```python
from build123d import *

# Parameters (mm, degrees)
SKETCH_1_W      = 40
SKETCH_1_H      = 40
EXTRUDE_1_DEPTH = 20
SKETCH_2_R      = 3
EXTRUDE_2_DEPTH = 4.5
SKETCH_4_R      = 2
SKETCH_4_W      = 8
SKETCH_4_H      = 20
EXTRUDE_4_DEPTH = 2.7
SKETCH_5_W      = 4
SKETCH_5_H      = 7
EXTRUDE_5_DEPTH = 7


with BuildPart() as part:
    # 草图1 → 凸台-拉伸1 (new body)
    with BuildSketch(Plane(origin=(0, 0, 0), x_dir=(1, 0, 0), z_dir=(0, 1, 0))):
        with Locations((20, 20)):
            Rectangle(SKETCH_1_W, SKETCH_1_H)
    extrude(amount=EXTRUDE_1_DEPTH)

    # 草图2 → 凸台-拉伸2 (add)
    with BuildSketch(Plane.XY):
        with Locations(Location((10, 10, 0), (0, 0, 180))):
            Circle(SKETCH_2_R)
    extrude(amount=EXTRUDE_2_DEPTH)

    # 草图4 → 凸台-拉伸4 (add)
    # profile 1 of 3: a face of its own
    with BuildSketch(Plane(origin=(0, 0, -12.3), x_dir=(-1, 0, 0), z_dir=(0, 0, -1))):
        with BuildLine():
            Line((-44.5, 17), (-44.5, 20))
            Line((-44.5, 20), (-48, 20))
            Line((-48, 20), (-48, 0))
            Line((-48, 0), (-40, 0))
            Line((-40, 0), (-40, 15))
            Line((-40, 15), (-42.5, 15))
            ThreePointArc((-42.5, 15), (-45.914213562, 13.585786438), (-44.5, 17))
        make_face()
        with Locations((-44.5, 5)):
            Circle(SKETCH_4_R, mode=Mode.SUBTRACT)
    # profile 2 of 3: a face of its own
    with BuildSketch(Plane(origin=(0, 0, -12.3), x_dir=(-1, 0, 0), z_dir=(0, 0, -1))):
        with BuildLine():
            Line((-40, 15), (-40, 20))
            Line((-40, 20), (-44.5, 20))
            Line((-44.5, 20), (-44.5, 17))
            ThreePointArc((-44.5, 17), (-43.085786438, 16.414213562), (-42.5, 15))
            Line((-42.5, 15), (-40, 15))
        make_face()
    # profile 3 of 3: a face of its own
    with BuildSketch(Plane(origin=(0, 0, -12.3), x_dir=(-1, 0, 0), z_dir=(0, 0, -1))):
        with Locations((4, 10)):
            Rectangle(SKETCH_4_W, SKETCH_4_H)
        with Locations((4.5, 5)):
            Circle(SKETCH_4_R, mode=Mode.SUBTRACT)
        with Locations((4.5, 15)):
            Circle(SKETCH_4_R, mode=Mode.SUBTRACT)
    extrude(amount=-EXTRUDE_4_DEPTH)

    # 草图5 → 凸台-拉伸5 (add)
    with BuildSketch(Plane.ZY):
        with Locations((-35, 10)):
            Rectangle(SKETCH_5_W, SKETCH_5_H)
    extrude(amount=EXTRUDE_5_DEPTH)


solid = part.part
```
The model under review builds one solid part; all positions refer to its coordinate system, in mm. A direction names the side the tool comes from. Coordinates: 2 decimals unless noted, no trailing zeros. Order: outer loops, then holes, each group sorted by start corner. A loop starts at its lowest first (then second) coordinate and runs counter-clockwise, first axis right, second up. Notation, with made-up numbers: M 36,-40 L 77,-40 A20 cw 77,-27 Z; hole C 68,-28.5 d6. An arc over 180 degrees is marked long. One line per question, with ' | ' between items.
(1) Add section C-C, the plane y = 18. Write out the cut boundary in (x, z).
Geometry results:
outline: M -8,-12.3 L 0,-12.3 L 0,-40 L 40,-40 L 40,-12.3 L 48,-12.3 L 48,-9.6 L 40,-9.6 L 40,0 L 0,0 L 0,-9.6 L -8,-9.6 Z
(2) Add section D-D, the plane z = -28. Write out the cut boundary in (x, y).
Geometry results:
outline: M 0,0 L 40,0 L 40,20 L 0,20 Z
(3) Add section B-B, the plane x = 10. Write out the cut boundary in (y, z).
Geometry results:
outline: M 0,-40 L 20,-40 L 20,0 L 13,0 L 13,4.5 L 7,4.5 L 7,0 L 0,0 Z
(4) The part is to be moulded in two halves that separate along Z. For faces 6 (the face through (20, 10, 0)), 7 (the face through (-4, 10, -12.3)), 8 (the face through (20, 20, -20)), say which applies: +Z half, -Z half, draft (parallel to the pull), parting line (faces both ways), or undercut.
Geometry results:
face 6: +Z half | face 7: undercut | face 8: draft
(5) Add section A-A, the plane y = 5. Write out the cut boundary in (x, z), then the cut area to 3 significant figures.
Geometry results:
outline: M -8,-12.3 L -6.5,-12.3 L -6.5,-9.6 L -8,-9.6 Z; M -2.5,-12.3 L 0,-12.3 L 0,-40 L 40,-40 L 40,-12.3 L 42.5,-12.3 L 42.5,-9.6 L 40,-9.6 L 40,0 L 0,0 L 0,-9.6 L -2.5,-9.6 Z; M 46.5,-12.3 L 48,-12.3 L 48,-9.6 L 46.5,-9.6 Z | area: 1,620 mm²
(6) For probe 1 along Y at (x, z) = (44.5, -10.6); probe 2 along Y at (x, z) = (-4, -10); probe 3 along X at (y, z) = (9.5, -1), list the stretches that pass through material, from the lowest coordinate up. Write a range as from..to.
Geometry results:
probe 1: y = 0..3, 7..13, 17..20 | probe 2: y = 0..3.06, 6.94..13.06, 16.94..20 | probe 3: x = 0..40
(7) Machinability: for faces 1 (the face through (-4.24, 16.983, -10.969)), 2 (the face through (0, 10, -5)), 3 (the face through (40, 10, -26)), 4 (the face through (-7, 10, -35)), 5 (the face through (44, 10, -9.6)), which of the approach directions +Z, -Z, +X, -X, +Y, -Y give a long, thin tool a straight path to every point of the face, cutting with its end or side? Answer none if there is none.
Geometry results:
face 1: +Z | face 2: +Z, -X, +Y, -Y | face 3: -Z, +X, +Y, -Y | face 4: -Z, -X, +Y, -Y | face 5: +Z, +X, +Y, -Y
(8) Insertion check: pin 1 (6 mm diameter, centred on x = 23, y = 12.5, fed in from +Z); pin 2 (7.5 mm diameter, centred on y = 5.5, z = -4, fed in from -X); pin 3 (3 mm diameter, centred on x = -2, y = 14.5, fed in from -Z). Each pin has a flat end and moves straight along its axis. Give the tip position at first contact, or say it passes through.
Geometry results:
pin 1: stops at z = 0 | pin 2: stops at x = 0 | pin 3: stops at z = -37
